Work out the finished part from the listing and answer in its coordinate system (mm). A direction names the side the tool comes from. Round coordinates to 2 decimals unless told otherwise and drop trailing zeros. Loops run counter-clockwise (first coordinate to the right, second up) from the corner with the lowest first, then second, coordinate; pieces in that order, holes last.
```python
from build123d import *

# Parameters (mm, degrees)
BOSS_EXTRUDE1_DEPTH = 38.1
SKETCH5_R           = 11.176
CUT_EXTRUDE1_DEPTH  = 38.1
FILLET1_R           = 15
SKETCH6_R           = 1.51
CUT_EXTRUDE2_DEPTH  = 10
SKETCH11_R          = 2.75
CUT_EXTRUDE5_DEPTH  = 5
SKETCH12_R          = 2.75
BOSS_EXTRUDE2_DEPTH = 3
SKETCH13_R          = 1.5
CUT_EXTRUDE6_DEPTH  = 3


with BuildPart() as part:
    # Sketch1 → Boss-Extrude1 (new body)
    with BuildSketch(Plane.XY):
        Polygon((-76.717654375, 44.038289207), (-0.517654375, 44.038289207), (-0.517654375, 4.028289207), (-6.105654375, 4.028289207), (-6.105654375, 39.588289207), (-71.129654375, 39.588289207), (-71.129654375, 4.028289207), (-76.717654375, 4.028289207), align=None)
    extrude(amount=BOSS_EXTRUDE1_DEPTH)

    # Sketch5 → Cut-Extrude1 (cut)
    with BuildSketch(Plane.ZY.offset(6.105654375)):
        with Locations((19.05, 21.178289207)):
            Circle(SKETCH5_R)
    cut_extrude1 = extrude(amount=-CUT_EXTRUDE1_DEPTH, mode=Mode.SUBTRACT)

    # Mirror3: Cut-Extrude1 across plane
    add(cut_extrude1.mirror(Plane.ZY.offset(38.617654375)), mode=Mode.SUBTRACT)

    # Fillet1
    fillet1_edges = [part.edges().sort_by_distance(p)[0] for p in [
        (-73.923654375, 4.028289207, 0),
        (-3.311654375, 4.028289207, 38.1),
        (-73.923654375, 4.028289207, 38.1),
        (-3.311654375, 4.028289207, 0),
    ]]
    fillet(fillet1_edges, radius=FILLET1_R)

    # Sketch6 → Cut-Extrude2 (cut)
    with BuildSketch(Plane(origin=(0, 44.038289207, 0), x_dir=(1, 0, 0), z_dir=(0, 1, 0))):
        with Locations((-56.617654375, -19.05)):
            Circle(SKETCH6_R)
        with Locations((-20.617654375, -19.05)):
            Circle(SKETCH6_R)
    extrude(amount=-CUT_EXTRUDE2_DEPTH, mode=Mode.SUBTRACT)

    # Sketch11 → Cut-Extrude5 (cut)
    with BuildSketch(Plane(origin=(0, 44.038289207, 0), x_dir=(1, 0, 0), z_dir=(0, 1, 0))):
        with Locations((-56.617654375, -19.05)):
            Circle(SKETCH11_R)
        with Locations((-20.617654375, -19.05)):
            Circle(SKETCH11_R)
    extrude(amount=-CUT_EXTRUDE5_DEPTH, mode=Mode.SUBTRACT)

    # Sketch12 → Boss-Extrude2 (add)
    with BuildSketch(Plane(origin=(0, 0, 0), x_dir=(-1, 0, 0), z_dir=(0, 0, -1))):
        with BuildLine():
            Line((6.105654375, 39.588289207), (71.129654375, 39.588289207))
            Line((71.129654375, 39.588289207), (71.129654375, 28.628518045))
            Line((71.129654375, 28.628518045), (65.259425536, 28.628518045))
            ThreePointArc((65.259425536, 28.628518045), (62.352582017, 29.420734639), (60.249654375, 31.578289207))
            ThreePointArc((60.249654375, 31.578289207), (59.564079492, 33.126822105), (57.949654375, 33.638289207))
            Line((57.949654375, 33.638289207), (19.045654375, 33.638289207))
            ThreePointArc((19.045654375, 33.638289207), (17.589014406, 33.034929176), (16.985654375, 31.578289207))
            ThreePointArc((16.985654375, 31.578289207), (14.882724316, 29.420741304), (11.975883214, 28.628527574))
            Line((11.975883214, 28.628527574), (6.105654375, 28.628527574))
            Line((6.105654375, 28.628527574), (6.105654375, 39.588289207))
        make_face()
        with Locations((65.009654375, 33.638289207)):
            Circle(SKETCH12_R, mode=Mode.SUBTRACT)
        with Locations((11.985654375, 33.638289207)):
            Circle(SKETCH12_R, mode=Mode.SUBTRACT)
    extrude(amount=-BOSS_EXTRUDE2_DEPTH)

    # Sketch13 → Cut-Extrude6 (cut)
    with BuildSketch(Plane.XY.offset(3)):
        with Locations((-28.497654375, 36.613289207)):
            Circle(SKETCH13_R)
        with Locations((-48.497654375, 36.613289207)):
            Circle(SKETCH13_R)
    extrude(amount=-CUT_EXTRUDE6_DEPTH, mode=Mode.SUBTRACT)


solid = part.part
```
1. Find section A-A (z = 19.05). Write down the section's boundary in (x, y), then the cut area to 3 significant figures.
Answer key:
outline: (-76.72, 4.03) - (-71.13, 4.03) - (-71.13, 10) - (-76.72, 10) - close; (-76.72, 32.35) - (-71.13, 32.35) - (-71.13, 39.59) - (-59.37, 39.59) - (-59.37, 44.04) - (-76.72, 44.04) - close; (-53.87, 39.59) - (-23.37, 39.59) - (-23.37, 44.04) - (-53.87, 44.04) - close; (-17.87, 39.59) - (-6.11, 39.59) - (-6.11, 32.35) - (-0.52, 32.35) - (-0.52, 44.04) - (-17.87, 44.04) - close; (-6.11, 4.03) - (-0.52, 4.03) - (-0.52, 10) - (-6.11, 10) - close
area: 438 mm2
2. Find section D-D (y = 8.5). Write down the section's boundary in (x, z), then the cut area to 3 significant figures.
Answer key:
outline: (-76.72, 4.32) - (-71.13, 4.32) - (-71.13, 33.78) - (-76.72, 33.78) - close; (-6.11, 4.32) - (-0.52, 4.32) - (-0.52, 33.78) - (-6.11, 33.78) - close
area: 329 mm2
3. Find section C-C (x = -53). Write down the section's boundary in (y, z).
Answer key:
outline: (33.64, 0) - (44.04, 0) - (44.04, 38.1) - (39.59, 38.1) - (39.59, 3) - (33.64, 3) - close
4. Given pin 1 (1.5 mm diameter, centred on x = -67.5, z = 2, fed in from -Y); pin 2 (7 mm diameter, centred on x = -56.62, z = 19.05, fed in from +Y); pin 3 (4 mm diameter, centred on x = -48.5, y = 36.61, fed in from +Z); pin 4 (1.5 mm diameter, centred on x = -29.5, z = 1, fed in from -Y), each flat-ended and moving along its own axis, determine where each tip first touches the part or whether it passes through.
Answer key:
pin 1: stops at y = 28.63
pin 2: stops at y = 44.04
pin 3: stops at z = 3
pin 4: stops at y = 33.64
5. Determine the mould class of faces 4 (the face through (-39, 44.038, 19)), 5 (the face through (-3.351, 8.539, 4.277)), 6 (the face through (-76.718, 33, 19)), 7 (the face through (-73.885, 11.263, 24.207)) for opening direction Y: +Y half, -Y half, draft (parallel to the pull), parting line (faces both ways), or undercut.
Answer key:
face 4: +Y half
face 5: -Y half
face 6: draft
face 7: undercut
6. Find section B-B (y = 23.5). Write down the section's boundary in (x, z), then the cut area to 3 significant figures.
Answer key:
outline: (-76.72, 0) - (-71.13, 0) - (-71.13, 8.12) - (-76.72, 8.12) - close; (-76.72, 29.98) - (-71.13, 29.98) - (-71.13, 38.1) - (-76.72, 38.1) - close; (-6.11, 0) - (-0.52, 0) - (-0.52, 8.12) - (-6.11, 8.12) - close; (-6.11, 29.98) - (-0.52, 29.98) - (-0.52, 38.1) - (-6.11, 38.1) - close
area: 181 mm2
7. Consider probe 1 along X at (y, z) = (13, 7); probe 2 along X at (y, z) = (42, 19); probe 3 along Y at (x, z) = (-3.75, 19.05). Determine where each line is inside the solid, lowest interval first.
Answer key:
probe 1: x = -76.72 to -71.13, -6.11 to -0.52
probe 2: x = -76.72 to -59.37, -53.87 to -23.37, -17.87 to -0.52
probe 3: y = 4.03 to 10, 32.35 to 44.04
8. Which of the six approach directions +Z, -Z, +X, -X, +Y, -Y give full straight-line access (tool end or side, diameter ignored) to faces 1 (the face through (-71.13, 30, 27)), 2 (the face through (-0.518, 33, 19)), 3 (the face through (-62.39, 29.4, 1.48))?
Answer key:
face 1: +Z, -Y
face 2: +Z, -Z, +X, +Y, -Y
face 3: +Z, -Z, -Y
